from build123d import *

# Parameters (mm, degrees)
BOSS_EXTRUDE1_DEPTH     = 402
BOSS_EXTRUDE2_DEPTH     = 969
CUT_EXTRUDE1_DEPTH      = 1960.325116763
FILLET1_R               = 500
CUT_EXTRUDE2_START      = 402
SKETCH4_W               = 150
SKETCH4_H               = 750
CUT_EXTRUDE2_DEPTH      = 20
SKETCH7_R               = 20
CUT_EXTRUDE3_DEPTH      = 20
SKETCH8_R               = 20
CUT_EXTRUDE4_DEPTH      = 20
BOSS_EXTRUDE3_START     = -10
BOSS_EXTRUDE3_DEPTH     = 215
FILLET2_R               = 20
CUT_EXTRUDE5_DEPTH      = 226
CUT_EXTRUDE5_DEPTH_BACK = 1960.325116812
SKETCH10_R              = 60
CHAMFER1_SIZE           = 50
CHAMFER1_SIZE2          = 41.954981559
FILLET3_R               = 20
SKETCH11_R              = 315
CUT_EXTRUDE6_DEPTH      = 66
CUT_EXTRUDE7_DEPTH      = 1960.325116812
CUT_EXTRUDE7_DEPTH_BACK = 1960.325116812
SKETCH12_W              = 640
SKETCH12_H              = 46


with BuildPart() as part:
    # Sketch1 → Boss-Extrude1 (new body)
    with BuildSketch(Plane(origin=(0, 0, 0), x_dir=(1, 0, 0), z_dir=(0, 1, 0))):
        with BuildLine():
            Line((1046.337061031, 577.858493981), (1016.667317849, 565.870736079))
            ThreePointArc((1016.667317849, 565.870736079), (522.188011035, 660.289732015), (66.74007867, 445.832480877))
            ThreePointArc((66.74007867, 445.832480877), (33.691690874, 412.919114907), (2.599998001, 378.151425458))
            ThreePointArc((2.599998001, 378.151425458), (1.291392319, 376.582813438), (0, 375))
            Line((0, 375), (0, -375))
            ThreePointArc((0, -375), (1.291392319, -376.582813438), (2.599998001, -378.151425458))
            ThreePointArc((2.599998001, -378.151425458), (33.691690874, -412.919114907), (66.74007867, -445.832480877))
            ThreePointArc((66.74007867, -445.832480877), (522.187167102, -660.28962537), (1016.665827322, -565.871556268))
            Line((1016.665827322, -565.871556268), (1046.335850828, -577.858620343))
            ThreePointArc((1046.335850828, -577.858620343), (1567, -0.000608391), (1046.337061031, 577.858493981))
        make_face()
    extrude(amount=BOSS_EXTRUDE1_DEPTH)

    # Sketch2 → Boss-Extrude2 (add)
    with BuildSketch(Plane(origin=(0, 0, 0), x_dir=(1, 0, 0), z_dir=(0, 1, 0))):
        with BuildLine():
            Line((144, 408), (1021.890739397, 408))
            ThreePointArc((1021.890739397, 408), (1127.956756575, 364.066017178), (1171.890739397, 258))
            Line((1171.890739397, 258), (1171.890739397, -163))
            ThreePointArc((1171.890739397, -163), (1108.332910914, -316.442171517), (954.890739397, -380))
            Line((954.890739397, -380), (854.68972927, -380))
            ThreePointArc((854.68972927, -380), (837.543301071, -388.875644347), (834.890739397, -408))
            Line((834.890739397, -408), (1171.890739397, -408))
            ThreePointArc((1171.890739397, -408), (1219.999604094, -395.667195333), (1256.24212417, -361.710742752))
            ThreePointArc((1256.24212417, -361.710742752), (1363.13459057, 62.465453501), (1195.440223215, 466.482834313))
            ThreePointArc((1195.440223215, 466.482834313), (833.097116799, 602.555696564), (446.106721665, 595.715763658))
            ThreePointArc((446.106721665, 595.715763658), (307.869625647, 548.008401888), (185.923871205, 467.294586118))
            ThreePointArc((185.923871205, 467.294586118), (161.31953374, 440.222630818), (144, 408))
        make_face()
    extrude(amount=BOSS_EXTRUDE2_DEPTH)

    # Sketch3 → Cut-Extrude1 (cut, through all)
    with BuildSketch(Plane.XY):
        Polygon((144, 402), (773.717295908, 969), (144, 969), align=None)
    extrude(amount=-CUT_EXTRUDE1_DEPTH, mode=Mode.SUBTRACT)

    # Fillet1
    fillet1_edges = [part.edges().sort_by_distance(p)[0] for p in [
        (773.717295908, 969, -509.514721406),
    ]]
    fillet(fillet1_edges, radius=FILLET1_R)

    # Sketch4 → Cut-Extrude2 (cut)
    with BuildSketch(Plane(origin=(0, 0, 0), x_dir=(1, 0, 0), z_dir=(0, 1, 0)).offset(CUT_EXTRUDE2_START)):
        with Locations((685, -20)):
            Rectangle(SKETCH4_W, SKETCH4_H)
    extrude(amount=-CUT_EXTRUDE2_DEPTH, mode=Mode.SUBTRACT)

    # Sketch7 → Cut-Extrude3 (cut)
    with BuildSketch(Plane(origin=(0, 402, 0), x_dir=(1, 0, 0), z_dir=(0, 1, 0))):
        with Locations(Location((50, 375, 0), (0, 0, 270))):
            Circle(SKETCH7_R)
        with Locations(Location((50, -375, 0), (0, 0, 270))):
            Circle(SKETCH7_R)
    extrude(amount=-CUT_EXTRUDE3_DEPTH, mode=Mode.SUBTRACT)

    # Sketch8 → Cut-Extrude4 (cut)
    with BuildSketch(Plane(origin=(0, 969, 0), x_dir=(1, 0, 0), z_dir=(0, 1, 0))):
        with Locations(Location((1213, 375, 0), (0, 0, 270))):
            Circle(SKETCH8_R)
        with Locations(Location((1213, -375, 0), (0, 0, 270))):
            Circle(SKETCH8_R)
    extrude(amount=-CUT_EXTRUDE4_DEPTH, mode=Mode.SUBTRACT)

    # Sketch9 → Boss-Extrude3 (add)
    with BuildSketch(Plane.XY.offset(BOSS_EXTRUDE3_START)):
        Polygon((0, 0), (357, 0), (357, -28), (-223, -28), (-223, 17), (-128, 17), (-128, 173), (-223, 173), (-223, 218), (0, 218), align=None)
    extrude(amount=-BOSS_EXTRUDE3_DEPTH)

    # Fillet2
    fillet2_edges = [part.edges().sort_by_distance(p)[0] for p in [
        (-223, -5.5, -10),
        (-223, 195.5, -10),
        (-223, -5.5, -225),
        (-223, 195.5, -225),
    ]]
    fillet(fillet2_edges, radius=FILLET2_R)

    # Sketch10 → Cut-Extrude5 (cut, two sides: drawn at the far end of the back side and taken through both)
    with BuildSketch(Plane(origin=(0, 0, 0), x_dir=(1, 0, 0), z_dir=(0, 1, 0)).offset(-CUT_EXTRUDE5_DEPTH_BACK)):
        with Locations(Location((-128, 117.5, 0), (0, 0, 270))):
            Circle(SKETCH10_R)
    extrude(amount=CUT_EXTRUDE5_DEPTH + CUT_EXTRUDE5_DEPTH_BACK, mode=Mode.SUBTRACT)

    # Chamfer1
    chamfer1_edges = [part.edges().sort_by_distance(p)[0] for p in [
        (0, 0, -300),
        (0, 0, 182.5),
    ]]
    chamfer1_side = [part.faces().sort_by_distance(p)[0] for p in [
        (765.492068196, 0, 5.511575813),
    ]]
    chamfer(chamfer1_edges, length=CHAMFER1_SIZE, length2=CHAMFER1_SIZE2, reference=chamfer1_side[0])

    # Fillet3
    fillet3_edges = [part.edges().sort_by_distance(p)[0] for p in [
        (0, 402, 0),
    ]]
    fillet(fillet3_edges, radius=FILLET3_R)

    # Sketch11 → Cut-Extrude6 (cut)
    with BuildSketch(Plane(origin=(0, 0, 0), x_dir=(1, 0, 0), z_dir=(0, 1, 0))):
        with Locations(Location((687, 0, 0), (0, 0, 270))):
            Circle(SKETCH11_R)
    extrude(amount=CUT_EXTRUDE6_DEPTH, mode=Mode.SUBTRACT)

    # Sketch12 → Cut-Extrude7 (cut, two sides: drawn at the far end of the back side and taken through both)
    with BuildSketch(Plane.XY.offset(-CUT_EXTRUDE7_DEPTH_BACK)):
        with Locations((692, 23)):
            Rectangle(SKETCH12_W, SKETCH12_H)
    extrude(amount=CUT_EXTRUDE7_DEPTH + CUT_EXTRUDE7_DEPTH_BACK, mode=Mode.SUBTRACT)


solid = part.part
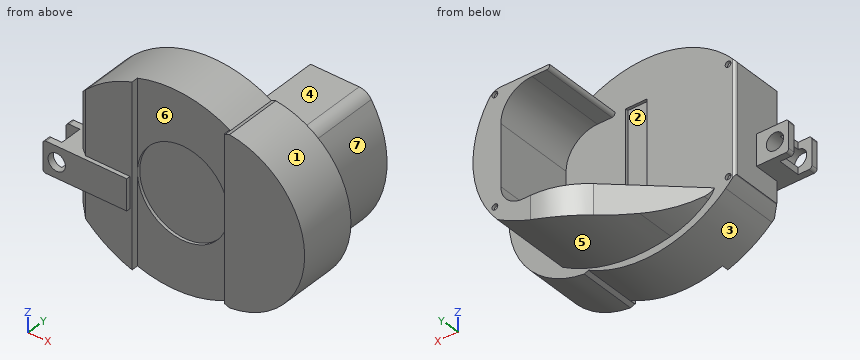
Part model, mm, in its own coordinate system. Face numbers are marked on the shaded views. A direction names the side the tool comes from. Give positions to 0.01 mm unless a question says otherwise; leave off trailing zeros. Loops run counter-clockwise (first coordinate to the right, second up) from the corner with the lowest first, then second, coordinate; pieces in that order, holes last. Notation, with made-up numbers: M 73.25,58 L 122.25,58 A24 cw 122.25,90 Z; hole C -35.5,12.25 d3. An arc over 180 degrees is marked long. Put each result on its own line as item: value. Start each with the question number.
1) Saw through at C-C (x = 422.5). List the corners of the cut face in (y, z).
2) 3-axis set-ups, long thin cutter, end or side, ignore diameter. For the marked faces 5, 6 and 7: which of +Z, -Z, +X, -X, +Y, -Y reach the whole face in a straight line?
3) Probe probe 1 along Z at (x, y) = (1213, 960); probe 2 along Y at (x, z) = (694.5, 585); probe 3 along Z at (x, y) = (1021, 814.5). List the from-to ranges inside material, lowest first.
4) Saw through at A-A (z = -117.5). State how many separate pieces and enclosed holes the cut face has, then the cut area to 3 significant figures.
5) Saw through at D-D (z = 46). List the corners of the cut face in (x, y), then the cut area to 3 significant figures.
6) Saw through at B-B (y = 586.5). List the corners of the cut face in (x, z).
7) Pull direction Z, two halves, no side cores. Call the marked faces 1, 2, 3 and 4: +Z half, -Z half, draft (parallel to the pull), parting line (faces both ways), or undercut.
8) Flat gauge pins, fed straight in: pin 1 (1.5 mm diameter, centred on x = 70.5, z = 171, fed in from -Y); pin 2 (10 mm diameter, centred on y = 393.5, z = 111, fed in from +X); pin 3 (1 mm diameter, centred on x = 789.5, z = -315, fed in from +Y). Where does each tip first touch, or does it go through?
Numbers:
1. outline: M 46,-641.32 L 402,-641.32 L 402,-590.26 L 652.76,-590.26 L 652.76,-408 L 402,-408 L 402,641.32 L 46,641.32 L 46,171.07 L 66,171.07 L 66,-171.07 L 46,-171.07 Z
2. face 5: -Z, +Y
2. face 6: +Z, -Z, -Y
2. face 7: +X, +Y
3. probe 1: -445.37 to -395, -355 to 355, 395 to 399.16
3. probe 2: 46 to 402
3. probe 3: -551.53 to -408, 369.68 to 408
4. separate pieces: 3
4. enclosed holes: 0
4. area: 716,000 mm^2
5. outline: M 0,41.95 L 50,0 L 372,0 L 372,46 L 375.38,46 L 375.38,66 L 998.62,66 L 998.62,46 L 1012,46 L 1012,0 L 1565.18,0 L 1565.18,402 L 1362.61,402 L 1362.61,969 L 1171.89,969 L 1171.89,402 L 760,402 L 760,382 L 610,382 L 610,402 L 20,402 A20 ccw 0,382 Z
5. area: 691,000 mm^2
6. outline: M 348.91,-566.33 A581 ccw 446.11,-595.72 A1033 ccw 1195.44,-466.48 A695 ccw 1256.24,361.71 A100 ccw 1171.89,408 L 834.89,408 A21 ccw 854.69,380 L 954.89,380 A217 cw 1171.89,163 L 1171.89,-258 A150 cw 1021.89,-408 L 348.91,-408 Z
7. face 1: parting line
7. face 2: undercut
7. face 3: -Z half
7. face 4: +Z half
8. pin 1: y = 0
8. pin 2: x = 1557.25
8. pin 3: y = 402
